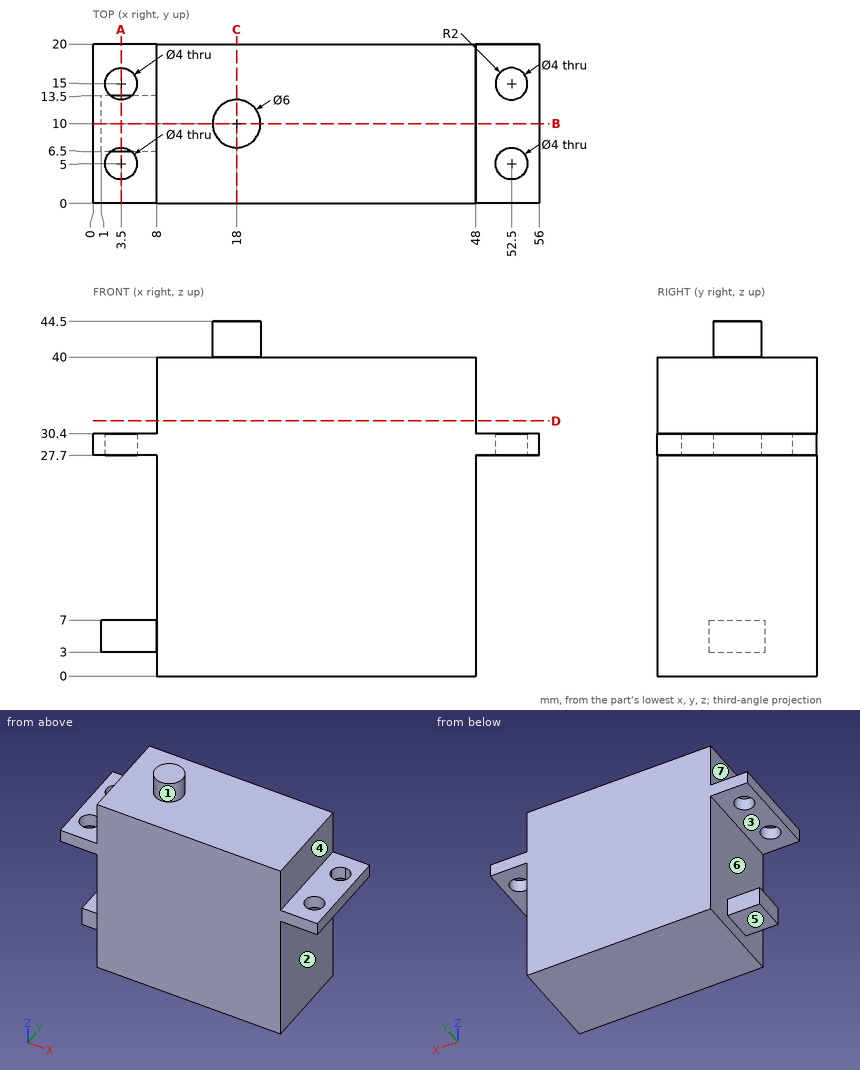
Study the drawing (mm; zero at the part's minimum x, y, z) and answer. A direction names the side the tool comes from. Give positions to 0.01 mm unless a question says otherwise; leave off trailing zeros. Order: outer loops, then holes, each group sorted by start corner. A loop starts at its lowest first (then second) coordinate and runs counter-clockwise, first axis right, second up. Notation, with made-up numbers: M -21.75,22 L 19.25,22 A31 ccw 19.25,53 Z; hole C -33,18.5 d5. An arc over 180 degrees is marked long. Put each result on its own line as item: value. Start each with the question number.
Item 1: The part is cut by section B-B, the plane y = 10. Determine the outline of the cut face in (x, z), and give its area (3 significant figures).
Item 2: The part is cut by section C-C, the plane x = 18. Determine the outline of the cut face in (y, z), and give its area (3 significant figures).
Item 3: Find the intervals of material crossed by line 1 along Y through (x, z) = (52, 28); line 2 along Z through (x, y) = (5.5, 13.25); line 3 along X through (y, z) = (3, 14), in increasing order.
Item 4: The part is cut by section A-A, the plane x = 3.5. Determine the outline of the cut face in (y, z).
Item 5: The part is cut by section D-D, the plane z = 32. Determine the outline of the cut face in (x, y).
Item 6: Which of the six approach directions +Z, -Z, +X, -X, +Y, -Y give full straight-line access (tool end or side, diameter ignored) to the marked faces 1, 2, 3 and 4?
Item 7: Flat-ended cylindrical pins translate along their axes: P1, Ø5, axis at y = 10, z = 35, coming from the -X side; P2, Ø7.5, axis at x = 3.5, y = 9, coming from the -Z side; P3, Ø4, axis at x = 51, y = 12, coming from the +Z side; P4, Ø3.5, axis at x = 52.5, y = 5, coming from the +Z side. Find the tip coordinate at first contact, or state that the pin passes through.
Item 8: For a pull along Z with two mould halves and no side action, classify the marked faces 5, 6 and 7 as +Z half, -Z half, draft (parallel to the pull), parting line (faces both ways), or undercut.
Answer key:
1. outline: M 0,27.7 L 8,27.7 L 8,7 L 1,7 L 1,3 L 8,3 L 8,0 L 48,0 L 48,27.7 L 56,27.7 L 56,30.4 L 48,30.4 L 48,40 L 21,40 L 21,44.5 L 15,44.5 L 15,40 L 8,40 L 8,30.4 L 0,30.4 Z
1. area: 1,700 mm²
2. outline: M 0,0 L 20,0 L 20,40 L 13,40 L 13,44.5 L 7,44.5 L 7,40 L 0,40 Z
2. area: 827 mm²
3. line 1: y = 0 to 3.06, 6.94 to 13.06, 16.94 to 20
3. line 2: z = 3 to 7, 27.7 to 30.4
3. line 3: x = 8 to 48
4. outline: M 0,27.7 L 3,27.7 L 3,30.4 L 0,30.4 Z; M 6.5,3 L 13.5,3 L 13.5,7 L 6.5,7 Z; M 7,27.7 L 13,27.7 L 13,30.4 L 7,30.4 Z; M 17,27.7 L 20,27.7 L 20,30.4 L 17,30.4 Z
5. outline: M 8,0 L 48,0 L 48,20 L 8,20 Z
6. face 1: +Z
6. face 2: -Z, +X, +Y, -Y
6. face 3: -X, +Y, -Y
6. face 4: +Z, +X, +Y, -Y
7. P1: stops at x = 8
7. P2: stops at z = 3
7. P3: stops at z = 30.4
7. P4: passes through
8. face 5: -Z half
8. face 6: undercut
8. face 7: draft
